The listing builds one solid part. Answer for the finished solid, in the listing's coordinates (mm). A direction names the side the tool comes from. Give positions to 0.01 mm unless a question says otherwise; leave off trailing zeros. Loops run counter-clockwise (first coordinate to the right, second up) from the corner with the lowest first, then second, coordinate; pieces in that order, holes last. Notation, with made-up numbers: M 68.5,56.5 L 109.5,56.5 A29 cw 109.5,86.5 Z; hole C 39,-2 d7. An arc over 180 degrees is marked long. One line per item, written item: value. Start each with the question number.
Q1. A cutting plane is placed at A-A, the plane z = 0. Determine the outline of the cut face in (x, y) (3 decimals), and give its area (3 significant figures).
Q2. The mould has two halves that part along Z. Classify faces 3 (the flat face through (8.738, -2.4, 2.4)), 4 (the cylindrical face through (8.419, 9.794, -2.175)), 5 (the cylindrical face through (3.87, 1.93, -2.52)): +Z half, -Z half, draft (parallel to the pull), parting line (faces both ways), or undercut.
Q3. Flat-ended cylindrical pins translate along their axes: pin 1 (0.5 mm diameter, centred on x = 2.5, y = 0, fed in from -Z); pin 2 (0.5 mm diameter, centred on x = 5.5, z = 0, fed in from -Y); pin 3 (1.5 mm diameter, centred on x = 4.5, y = 4.5, fed in from -Z); pin 4 (5.5 mm diameter, centred on y = 0, z = 0, fed in from -X). Find the tip coordinate at first contact, or state that the pin passes through.
Q4. For faces 1 (the cylindrical face through (-0.833, 9.794, -2.175)), 2 (the flat face through (0.114, 7, -2)), determine the directions among +Z, -Z, +X, -X, +Y, -Y from which every point of the face is accessible in a straight line to the end or side of a thin tool.
Q5. Consider L1, parallel to Z at x = 5.75, y = 0.25; L2, parallel to Y at x = 5.75, z = 0 (3 decimals); L3, parallel to X at y = 8, z = -0.5. Determine where each line is inside the solid, lowest interval first.
from build123d import *

# Parameters (mm, degrees)
SKETCH4_R          = 7.7597
SKETCH4_R_2        = 7.60095
CUT_EXTRUDE2_DEPTH = 7.366
CUT_EXTRUDE1_DEPTH = 7.366
CIRPATTERN1_COUNT  = 24
SKETCH6_R          = 1.4605
CUT_EXTRUDE3_DEPTH = 17.66336796
CUT_EXTRUDE4_DEPTH = 1.016
CIRPATTERN2_COUNT  = 2
CIRPATTERN2_ANGLE  = 90
CIRPATTERN3_COUNT  = 2
CIRPATTERN3_ANGLE  = 90
SKETCH9_W          = 8.047950053
SKETCH9_H          = 15.828316952
CUT_EXTRUDE5_DEPTH = 7.62


with BuildPart() as part:
    # Sketch1 → Revolve1 (revolve)
    with BuildSketch(Plane.XY, mode=Mode.PRIVATE) as revolve1_sk:
        with BuildLine():
            Line((-8.7376, 3.175), (8.7376, 3.175))
            Line((8.7376, 3.175), (8.7376, 10.033))
            Line((8.7376, 10.033), (8.10895, 10.033))
            ThreePointArc((8.10895, 10.033), (7.642486723, 9.238300334), (7.4803, 8.3312))
            Line((7.4803, 8.3312), (7.4803, 7.7597))
            Line((7.4803, 7.7597), (0.1143, 7.7597))
            Line((0.1143, 7.7597), (0.1143, 8.3312))
            ThreePointArc((0.1143, 8.3312), (-0.047886723, 9.238300334), (-0.51435, 10.033))
            Line((-0.51435, 10.033), (-1.143, 10.033))
            Line((-1.143, 10.033), (-1.143, 5.6134))
            Line((-1.143, 5.6134), (-8.7376, 5.6134))
            Line((-8.7376, 5.6134), (-8.7376, 3.175))
        make_face()
    revolve(revolve1_sk.sketch.rotate(Axis((-8.7376, 0, 0), (1, 0, 0)), 90), axis=Axis((-8.7376, 0, 0), (1, 0, 0)))

    # Sketch4 → Cut-Extrude2 (cut)
    with BuildSketch(Plane(origin=(0.1143, 0, 0), x_dir=(0, 0, -1), z_dir=(1, 0, 0))):
        Circle(SKETCH4_R)
        Circle(SKETCH4_R_2, mode=Mode.SUBTRACT)
    extrude(amount=CUT_EXTRUDE2_DEPTH, mode=Mode.SUBTRACT)

    # Sketch3 → Cut-Extrude1 (cut)
    with BuildSketch(Plane(origin=(0.1143, 0, 0), x_dir=(0, 0, -1), z_dir=(1, 0, 0))):
        with BuildLine():
            Line((-0.643066132, 7.57369836), (-0.340952079, 6.925812683))
            Line((-0.340952079, 6.925812683), (0.340952079, 6.925812683))
            Line((0.340952079, 6.925812683), (0.643066132, 7.57369836))
            ThreePointArc((0.643066132, 7.57369836), (0, 7.60095), (-0.643066132, 7.57369836))
        make_face()
    cut_extrude1 = extrude(amount=CUT_EXTRUDE1_DEPTH, mode=Mode.SUBTRACT)

    # CirPattern1: Cut-Extrude1 ×24 about axis
    cirpattern1_axis = Axis((0, 0, 0), (1, 0, 0))
    for i in range(1, CIRPATTERN1_COUNT):
        add(cut_extrude1.rotate(cirpattern1_axis, i * 360 / CIRPATTERN1_COUNT), mode=Mode.SUBTRACT)

    # Sketch6 → Cut-Extrude3 (cut, through all)
    with BuildSketch(Plane(origin=(0, 0, 0), x_dir=(1, 0, 0), z_dir=(0, 1, 0))):
        with Locations(Location((-4.9403, 0, 0), (0, 0, 90))):
            Circle(SKETCH6_R)
    cut_extrude3 = extrude(amount=CUT_EXTRUDE3_DEPTH, mode=Mode.SUBTRACT)

    # CirPattern2: Cut-Extrude3 ×2 about axis
    cirpattern2_axis = Axis((-8.7376, 0, 0), (1, 0, 0))
    for i in range(1, CIRPATTERN2_COUNT):
        add(cut_extrude3.rotate(cirpattern2_axis, i * CIRPATTERN2_ANGLE / (CIRPATTERN2_COUNT - 1)), mode=Mode.SUBTRACT)


with BuildPart() as body_2:
    # Sketch7 → Revolve2 (revolve)
    with BuildSketch(Plane.XY, mode=Mode.PRIVATE) as revolve2_sk:
        Polygon((-6.1087, 5.6134), (-4.9403, 5.6134), (-4.9403, 3.556), (-6.1087, 3.556), (-6.3627, 3.81), (-6.3627, 5.3594), align=None)
    revolve(revolve2_sk.sketch.rotate(Axis((-4.9403, 3.556, 0), (0, 1, 0)), 270), axis=Axis((-4.9403, 3.556, 0), (0, 1, 0)))

    # Sketch8 → Cut-Extrude4 (cut)
    with BuildSketch(Plane(origin=(0, 5.6134, 0), x_dir=(1, 0, 0), z_dir=(0, 1, 0))):
        Polygon((-4.9403, 0.821223023), (-5.6515, 0.410611511), (-5.6515, -0.410611511), (-4.9403, -0.821223023), (-4.2291, -0.410611511), (-4.2291, 0.410611511), align=None)
    extrude(amount=-CUT_EXTRUDE4_DEPTH, mode=Mode.SUBTRACT)


with BuildPart() as cirpattern3_1:
    # CirPattern3: pattern copy
    add(body_2.part.rotate(Axis((0, 0, 0), (1, 0, 0)), 1 * CIRPATTERN3_ANGLE / (CIRPATTERN3_COUNT - 1)))


with BuildPart() as cut_extrude5_tool:
    # Sketch9 → Cut-Extrude5 (new, symmetric)
    with BuildSketch(Plane(origin=(0, 0, 0), x_dir=(1, 0, 0), z_dir=(0, 1, 0))):
        with Locations((-5.166975027, 0.16569051)):
            Rectangle(SKETCH9_W, SKETCH9_H)
    extrude(amount=CUT_EXTRUDE5_DEPTH, both=True)


with BuildPart() as part_1:
    add(part.part)

    # Cut-Extrude5: cut by cut_extrude5_tool
    add(cut_extrude5_tool.part, mode=Mode.SUBTRACT)


with BuildPart() as body_2_1:
    add(body_2.part)

    # Cut-Extrude5: cut by cut_extrude5_tool
    add(cut_extrude5_tool.part, mode=Mode.SUBTRACT)


with BuildPart() as cirpattern3_1_1:
    add(cirpattern3_1.part)

    # Cut-Extrude5: cut by cut_extrude5_tool
    add(cut_extrude5_tool.part, mode=Mode.SUBTRACT)


solid = part_1.part
Answer block:
1. outline: M -1.143,-10.033 L -0.514,-10.033 A2.618 ccw 0.114,-8.331 L 0.114,-6.926 L 7.48,-6.926 L 7.48,-8.331 A2.618 ccw 8.109,-10.033 L 8.738,-10.033 L 8.738,-3.175 L -1.143,-3.175 Z; M -1.143,3.175 L 8.738,3.175 L 8.738,10.033 L 8.109,10.033 A2.618 ccw 7.48,8.331 L 7.48,6.926 L 0.114,6.926 L 0.114,8.331 A2.618 ccw -0.514,10.033 L -1.143,10.033 Z
1. area: 88.4 mm^2
2. face 3: draft
2. face 4: parting line
2. face 5: undercut
3. pin 1: z = -6.93
3. pin 2: y = -6.93
3. pin 3: z = -6.24
3. pin 4: through
4. face 1: +X, -X
4. face 2: none
5. L1: -6.93 to -3.17, 3.17 to 6.93
5. L2: -6.926 to -3.175, 3.175 to 6.926
5. L3: -1.14 to 0.11, 7.48 to 8.74
